from build123d import *

# Parameters (mm, degrees)
BOSS_EXTRUDE1_DEPTH = 40.64
SKETCH6_R           = 1.1303
CUT_EXTRUDE1_DEPTH  = 158.779215984
SKETCH7_R           = 19.05
CUT_EXTRUDE2_DEPTH  = 158.779215984


with BuildPart() as part:
    # Sweep3: sweep along a path in Sketch2
    with BuildLine(Plane.XY) as sweep3_path:
        Line((-111.378641457, -46.568583299), (-11.322173751, -64.21123815))
        ThreePointArc((-11.322173751, -64.21123815), (49.947476571, -41.910909169), (61.269650322, 22.300328981))
        Line((61.269650322, 22.300328981), (48.238682861, 58.102617833))
    # 3DSketch1 → Sweep3 (sweep)
    with BuildSketch(Plane(origin=(-117.024291009, -78.586652965, -20.32), x_dir=(0.051794909001673446, 0.2937435257699459, 0.9544799780350292), z_dir=(0.984807753012208, -0.17364817766693055, 0))):
        Polygon((0, 0), (3.788092413, -12.121895721), (42.57815872, 0), (38.790066307, 12.121895721), align=None)
    sweep(path=sweep3_path.line)

    # Sketch5 → Boss-Extrude1 (add)
    with BuildSketch(Plane.XY.offset(20.32)):
        with BuildLine():
            Line((-16.967823303, -96.229307816), (-117.024291009, -78.586652965))
            Line((-117.024291009, -78.586652965), (-117.024291009, -97.7138))
            Line((-117.024291009, -97.7138), (-1.15e-07, -97.7138))
            ThreePointArc((-1.15e-07, -97.7138), (-8.516318873, -97.341969485), (-16.967823303, -96.229307816))
        make_face()
        with BuildLine():
            ThreePointArc((97.7138, 1.15e-07), (69.094090596, -69.094090596), (-1.15e-07, -97.7138))
            Line((-1.15e-07, -97.7138), (97.7138, -97.7138))
            Line((97.7138, -97.7138), (97.7138, 1.15e-07))
        make_face()
        with BuildLine():
            ThreePointArc((91.820936809, 33.420087881), (96.229307806, 16.96782336), (97.7138, 1.15e-07))
            Line((97.7138, 1.15e-07), (97.7138, 69.222376733))
            Line((97.7138, 69.222376733), (78.789969348, 69.222376733))
            Line((78.789969348, 69.222376733), (91.820936809, 33.420087881))
        make_face()
    extrude(amount=-BOSS_EXTRUDE1_DEPTH)

    # Sketch6 → Cut-Extrude1 (cut, through all)
    with BuildSketch(Plane.XY.offset(20.32)):
        with Locations((91.3638, -91.3638)):
            Circle(SKETCH6_R)
        with Locations((-41.9735, -91.3638)):
            Circle(SKETCH6_R)
    extrude(amount=-CUT_EXTRUDE1_DEPTH, mode=Mode.SUBTRACT)

    # Sketch7 → Cut-Extrude2 (cut, through all)
    with BuildSketch(Plane.XY.offset(20.32)):
        with Locations((-117.024291009, -97.7138)):
            Circle(SKETCH7_R)
    extrude(amount=-CUT_EXTRUDE2_DEPTH, mode=Mode.SUBTRACT)


solid = part.part
Geometry: final body of the model. Coordinates: model frame, mm. A direction names the side the tool comes from. Give positions to 0.01 mm unless a question says otherwise; leave off trailing zeros. Order: outer loops, then holes, each group sorted by start corner. A loop starts at its lowest first (then second) coordinate and runs counter-clockwise, first axis right, second up. Notation, with made-up numbers: (70, 63) -> (85, 63) arc R22 cw to (85, 96) -> close; hole circle Ø10 at (76, 88.25). An arc over 180 degrees is marked (long way). Put each result on its own line as item: value.
Q1. Section C-C, the plane x = 45. Return loops of the section in (y, z).
Here are the results:
outline: (-97.71, -20.32) -> (-72.13, -20.32) -> (-72.13, 20.32) -> (-97.71, 20.32) -> close
Q2. Section A-A, the plane z = 14. Return loops of the section in (x, y), then the cut area to 3 significant figures.
Here are the results:
outline: (-117.02, -78.66) arc R19.05 cw to (-97.97, -97.71) -> (97.71, -97.71) -> (97.71, 69.22) -> (78.79, 69.22) -> (66.86, 64.88) -> (79.89, 29.08) arc R85.01 cw to (-14.76, -83.72) -> (-114.82, -66.08) -> (-117.02, -78.59) -> close; hole circle Ø2.26 at (-41.97, -91.36); hole circle Ø2.26 at (91.36, -91.36)
area: 7,510 mm^2
Q3. Section B-B, the plane y = 42.5. Return loops of the section in (x, z).
Here are the results:
outline: (75, -20.32) -> (97.71, -20.32) -> (97.71, 20.32) -> (75, 20.32) -> close
Q4. Material intervals for L1, parallel to Y at x = 2, z = 12; L2, parallel to X at y = 0.5, z = 16.5; L3, parallel to Y at x = -52, z = 2.5, sorted ascending.
Here are the results:
L1: y = -97.71 to -84.99
L2: x = 85.01 to 97.71
L3: y = -97.71 to -77.16
Q5. Section D-D, the plane y = -8. Return loops of the section in (x, z).
Here are the results:
outline: (84.64, -20.32) -> (97.71, -20.32) -> (97.71, 20.32) -> (84.64, 20.32) -> close
Q6. Draft query along X for faces 4 (the face through (-103.4, -84.4, 0.3)), 5 (the face through (97.714, -15, 0)), 6 (the face through (64.32, -55.59, 0.28)). Return one class per face: released by +X, released by -X, zero draft, split by the parting line, or undercut.
Here are the results:
face 4: released by -X
face 5: released by +X
face 6: undercut
Q7. Reachability of faces 1 (the face through (73.28, 47.23, -0.28)), 2 (the face through (-115.937, -72.421, 0.284)), 3 (the face through (-64.09, -75.024, -0.284)) from +Z, -Z, +X, -X, +Y, -Y: full face, straight path, thin tool, end or side. Return the list, or none.
Here are the results:
face 1: +Z, -Z, -X
face 2: +Z, -Z, -X, +Y
face 3: +Z, -Z, +Y
Q8. Pin query (flat end, axial travel): pin 1 (2 mm diameter, centred on x = -84, z = 3, fed in from +Y); pin 2 (1.4 mm diameter, centred on x = -41.97, y = -91.36, fed in from -Z); pin 3 (12 mm diameter, centred on x = 71.5, z = -6, fed in from +Y); pin 4 (4 mm diameter, centred on y = 14, z = -13, fed in from -X). Return the tip coordinate at first contact, or that it passes through.
Here are the results:
pin 1: stops at y = -71.34
pin 2: passes through
pin 3: stops at y = 68.75
pin 4: stops at x = 83.49
